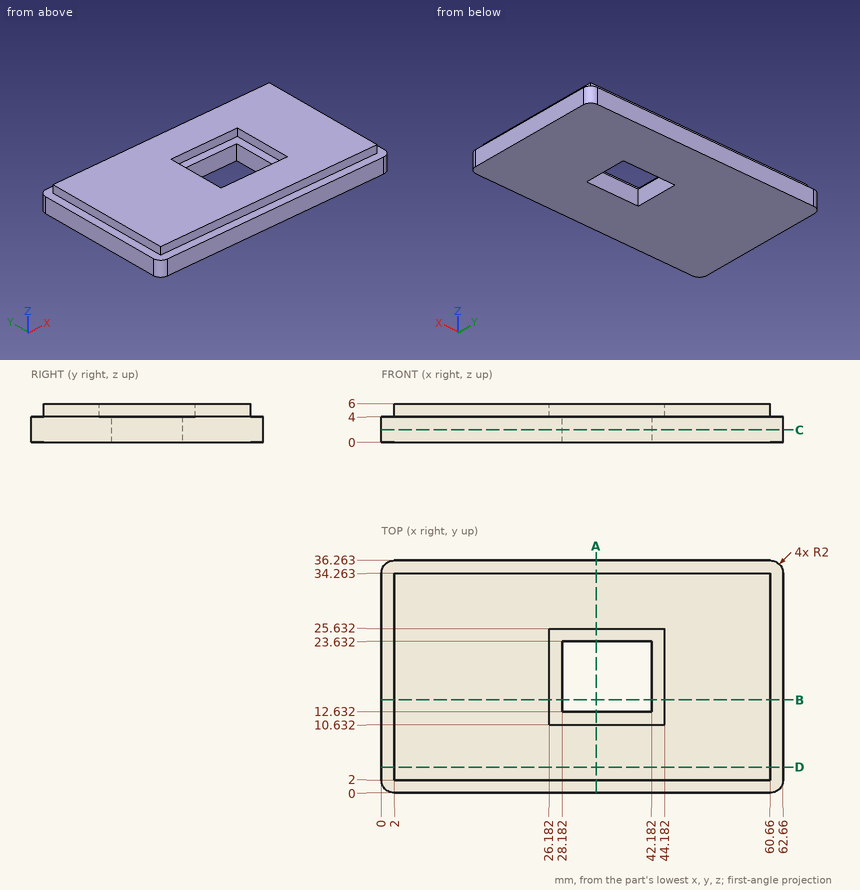
Check sheet for the drawn part. Datum: minimum x, y, z corner. Units: mm. Round coordinates to 2 decimals unless told otherwise and drop trailing zeros. Write each loop counter-clockwise with the first axis right and the second up, starting at its lowest first coordinate (ties: lowest second). Pieces come first, ordered by that corner, then holes. Notation, with made-up numbers: (71, -2) - (101, -2) arc R19 ccw to (101, 18) - close; hole circle Ø8 at (82.5, 11.5). An arc over 180 degrees is marked (long way). Write each question's results on one line, items separated by ' | '.
(1) Sectioned sample at B-B, the plane y = 14.5. Enter the section's corners in (x, z).
Computed:
outline: (0, 0) - (28.18, 0) - (28.18, 4) - (26.18, 4) - (26.18, 6) - (2, 6) - (2, 4) - (0, 4) - close; (42.18, 0) - (62.66, 0) - (62.66, 4) - (60.66, 4) - (60.66, 6) - (44.18, 6) - (44.18, 4) - (42.18, 4) - close
(2) Sectioned sample at A-A, the plane x = 33.5. Enter the section's corners in (y, z), plus the area to 3 significant figures.
Computed:
outline: (0, 0) - (12.63, 0) - (12.63, 4) - (10.63, 4) - (10.63, 6) - (2, 6) - (2, 4) - (0, 4) - close; (23.63, 0) - (36.26, 0) - (36.26, 4) - (34.26, 4) - (34.26, 6) - (25.63, 6) - (25.63, 4) - (23.63, 4) - close | area: 136 mm^2
(3) Depth check by flat-ended pin: pin 1 Ø2 at (x, z) = (37, 4.5) entering from +Y; pin 2 Ø1.6 at (y, z) = (25.5, 5) entering from +X; pin 3 Ø2 at (y, z) = (10.5, 5.5) entering from -X; pin 4 Ø2 at (x, z) = (40.5, 5.5) entering from +Y. Enter the tip coordinate at first touch or a pass-through.
Computed:
pin 1: stops at y = 36.26 | pin 2: stops at x = 60.66 | pin 3: stops at x = 2 | pin 4: stops at y = 34.26
(4) Sectioned sample at D-D, the plane y = 4. Enter the section's corners in (x, z).
Computed:
outline: (0, 0) - (62.66, 0) - (62.66, 4) - (60.66, 4) - (60.66, 6) - (2, 6) - (2, 4) - (0, 4) - close
(5) Thickness scan on probe 1 along X at (y, z) = (15, 3.25); probe 2 along X at (y, z) = (23.5, 4.35); probe 3 along Y at (x, z) = (40, 3.05). Record the ranges inside material, lowest first. Write a range as from..to.
Computed:
probe 1: x = 0..28.18, 42.18..62.66 | probe 2: x = 2..26.18, 44.18..60.66 | probe 3: y = 0..12.63, 23.63..36.26
(6) Sectioned sample at C-C, the plane z = 1.95. Enter the section's corners in (x, y).
Computed:
outline: (0, 2) arc R2 ccw to (2, 0) - (60.66, 0) arc R2 ccw to (62.66, 2) - (62.66, 34.26) arc R2 ccw to (60.66, 36.26) - (2, 36.26) arc R2 ccw to (0, 34.26) - close; hole (28.18, 12.63) - (42.18, 12.63) - (42.18, 23.63) - (28.18, 23.63) - close
